Could you check a few things on this model? Use its own coordinates, in mm. Face numbers are marked on the shaded views. A direction names the side the tool comes from. Coordinates: 2 decimals unless noted, no trailing zeros. Order: outer loops, then holes, each group sorted by start corner. A loop starts at its lowest first (then second) coordinate and runs counter-clockwise, first axis right, second up. Notation, with made-up numbers: (-6, -7.75) - (48, -7.75) arc R24 cw to (48, 20.25) - close; hole circle Ø10 at (21, 45.5). An arc over 180 degrees is marked (long way). One line per item, written item: value.
from build123d import *

# Parameters (mm, degrees)
F0_W     = 120
F0_H     = 65
F1_DEPTH = 50
F2_T     = -2.54
F3_R     = 3
F4_R     = 3


with BuildPart() as f1:
    # F0 (on Top) → F1 (new body)
    with BuildSketch(Plane.XY):
        Rectangle(F0_W, F0_H)
    extrude(amount=F1_DEPTH)

    # F2
    f2_openings = [f1.faces().sort_by_distance(p)[0] for p in [
        (0, 0, 0),
    ]]
    offset(amount=F2_T, openings=f2_openings)

    # F3
    f3_edges = [f1.edges().sort_by_distance(p)[0] for p in [
        (0, -32.5, 50),
        (60, 0, 50),
        (0, 32.5, 50),
        (-60, 0, 50),
        (-60, 32.5, 25),
        (60, 32.5, 25),
        (60, -32.5, 25),
        (-60, -32.5, 25),
    ]]
    fillet(f3_edges, radius=F3_R)

    # F4
    f4_edges = [f1.edges().sort_by_distance(p)[0] for p in [
        (0, 29.96, 47.46),
        (-57.46, 0, 47.46),
        (0, -29.96, 47.46),
        (57.46, 0, 47.46),
        (57.46, -29.96, 23.73),
        (57.46, 29.96, 23.73),
        (-57.46, 29.96, 23.73),
        (-57.46, -29.96, 23.73),
    ]]
    fillet(f4_edges, radius=F4_R)


solid = f1.part
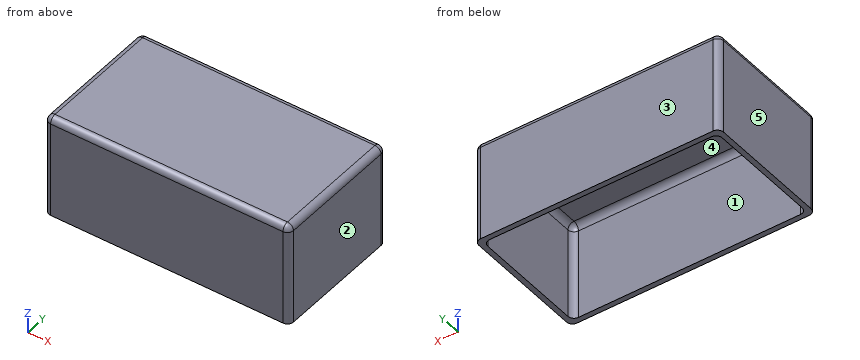
Item 1: I want a section at B-B on x = -2. Please give me the cut outline in (y, z), then the cut area to 3 significant figures.
Conclusion:
outline: (-32.5, 0) - (-29.96, 0) - (-29.96, 44.46) arc R3 cw to (-26.96, 47.46) - (26.96, 47.46) arc R3 cw to (29.96, 44.46) - (29.96, 0) - (32.5, 0) - (32.5, 47) arc R3 ccw to (29.5, 50) - (-29.5, 50) arc R3 ccw to (-32.5, 47) - close
area: 406 mm²
Item 2: I'm going to push a flat-ended pin straight in: pin 1 Ø5 at (x, y) = (9, 0.5) entering from -Z. Where does the tip first touch, or does it pass through?
Conclusion:
pin 1: z = 47.46
Item 3: For the marked faces 1 and 2, which set-ups out of +Z, -Z, +X, -X, +Y, -Y let a thin tool reach every point of the face, with its end or its side?
Conclusion:
face 1: -Z
face 2: +Z, -Z, +X, +Y, -Y
Item 4: Thinking about a two-plate mould opening in X: for the marked faces 3, 4 and 5, which applies, pulls with the +X half, pulls with the -X half, needs draft (parallel to the pull), parting line crosses it, or undercut?
Conclusion:
face 3: needs draft
face 4: undercut
face 5: pulls with the -X half
Item 5: I want a section at A-A on z = 14.5. Please give me the cut outline in (x, y), then the cut area to 3 significant figures.
Conclusion:
outline: (-60, -29.5) arc R3 ccw to (-57, -32.5) - (57, -32.5) arc R3 ccw to (60, -29.5) - (60, 29.5) arc R3 ccw to (57, 32.5) - (-57, 32.5) arc R3 ccw to (-60, 29.5) - close; hole (-57.46, -26.96) arc R3 ccw to (-54.46, -29.96) - (54.46, -29.96) arc R3 ccw to (57.46, -26.96) - (57.46, 26.96) arc R3 ccw to (54.46, 29.96) - (-54.46, 29.96) arc R3 ccw to (-57.46, 26.96) - close
area: 914 mm²
Item 6: If I drill on probe 1 along Y at (x, z) = (44, 26.5); probe 2 along X at (y, z) = (-20.5, 29); probe 3 along Z at (x, y) = (1.5, 26.5), over which ranges is the centre line in solid material (lowest first)?
Conclusion:
probe 1: -32.5 to -29.96, 29.96 to 32.5
probe 2: -60 to -57.46, 57.46 to 60
probe 3: 47.46 to 50
Item 7: I want a section at C-C on y = 11. Please give me the cut outline in (x, z), then the cut area to 3 significant figures.
Conclusion:
outline: (-60, 0) - (-57.46, 0) - (-57.46, 44.46) arc R3 cw to (-54.46, 47.46) - (54.46, 47.46) arc R3 cw to (57.46, 44.46) - (57.46, 0) - (60, 0) - (60, 47) arc R3 ccw to (57, 50) - (-57, 50) arc R3 ccw to (-60, 47) - close
area: 546 mm²
